Drawing for the job (mm, zero at the part's lowest x, y, z). Give positions to 0.01 mm unless a question says otherwise; leave off trailing zeros. Write each loop counter-clockwise with the first axis right and the second up, starting at its lowest first coordinate (ties: lowest second). Pieces come first, ordered by that corner, then holes.
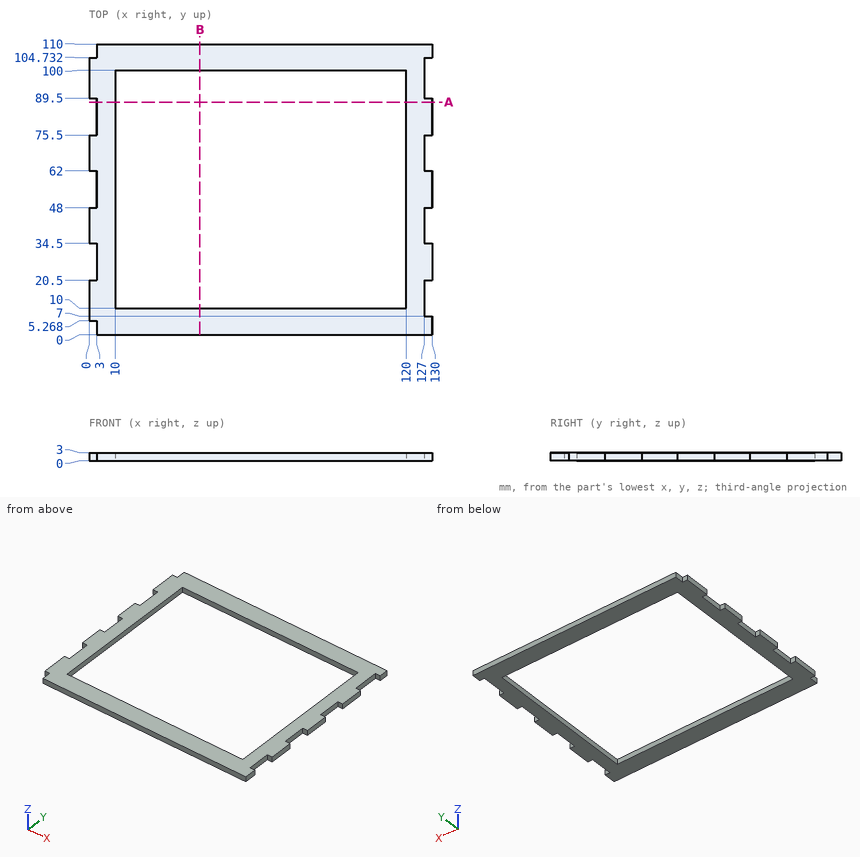
1. Probe probe 1 along Y at (x, z) = (18.5, 2.45); probe 2 along X at (y, z) = (93, 2.4); probe 3 along X at (y, z) = (27, 2.45). List the from-to ranges inside material, lowest first.
Calculated:
probe 1: y = 0 to 10, 100 to 110
probe 2: x = 0 to 10, 120 to 127
probe 3: x = 3 to 10, 120 to 130
2. Pin check, flat tip, straight feed: P1, Ø1.5, axis at y = 26, z = 2, coming from the -X side. Stop position of the tip, or through.
Calculated:
P1: stops at x = 3
3. Slice it at A-A, the plane y = 88. Write the cut outline in (x, z), and give its area (3 significant figures).
Calculated:
outline: (3, 0) - (10, 0) - (10, 3) - (3, 3) - close; (120, 0) - (130, 0) - (130, 3) - (120, 3) - close
area: 51.0 mm2
4. Slice it at B-B, the plane x = 42. Write the cut outline in (y, z).
Calculated:
outline: (0, 0) - (10, 0) - (10, 3) - (0, 3) - close; (100, 0) - (110, 0) - (110, 3) - (100, 3) - close
